Here's how the part is built. I have some questions about the finished solid (model axes, mm). Round coordinates to 2 decimals unless told otherwise and drop trailing zeros. Order: outer loops, then holes, each group sorted by start corner. A loop starts at its lowest first (then second) coordinate and runs counter-clockwise, first axis right, second up. Notation, with made-up numbers: M -20.5,11.5 L 30.5,11.5 A26 ccw 30.5,31.5 Z; hole C -1,-22.5 d10. An arc over 180 degrees is marked long. Write item = value, one per line. Start each with the question number.
Item 1: Please list where these lines run through material, in increasing order: L1, parallel to X at y = 6.5, z = 11.5; L2, parallel to Z at x = 99.5, y = 1; L3, parallel to Y at x = 84.5, z = 0.
Item 2: We'd pull the mould along Y, two halves only. Please class faces 1 (the face through (137.69, -9.76, 2.17)), 2 (the face through (10, -10, -3)): pulls with the +Y half, pulls with the -Y half, needs draft (parallel to the pull), parting line crosses it, or undercut.
Item 3: I want a section at A-A, the plane y = 0. List the corners of the cut face in (x, z) for me.
Item 4: I want a section at B-B, the plane x = 226. List the corners of the cut face in (y, z) for me.
Item 5: I'm going to push flat-ended pins straight in: P1, Ø2, axis at x = 0.5, y = -0.5, coming from the -Z side; P2, Ø8, axis at x = 167, y = -4, coming from the -Z side; P3, Ø5, axis at x = 228.5, z = 4.5, coming from the -Y side. Where does each tip first touch, or does it pass through?
```python
from build123d import *

# Parameters (mm, degrees)
SKETCH1_R           = 15
SKETCH1_R_2         = 10
BOSS_EXTRUDE1_DEPTH = 10
SKETCH1_2_R         = 10
BOSS_EXTRUDE2_DEPTH = 270
CHAMFER1_SIZE       = 1
FILLET1_R           = 1.5
SKETCH2_W           = 3
SKETCH2_H           = 32.549334764
CUT_EXTRUDE1_DEPTH  = 2


with BuildPart() as part:
    # Sketch1 → Boss-Extrude1 (new body)
    with BuildSketch(Plane(origin=(0, 0, 0), x_dir=(0, 0, -1), z_dir=(1, 0, 0))):
        Circle(SKETCH1_R)
        Circle(SKETCH1_R_2, mode=Mode.SUBTRACT)
    extrude(amount=BOSS_EXTRUDE1_DEPTH)

    # Sketch1<2> → Boss-Extrude2 (add)
    with BuildSketch(Plane(origin=(0, 0, 0), x_dir=(0, 0, -1), z_dir=(1, 0, 0))):
        Circle(SKETCH1_2_R)
    extrude(amount=BOSS_EXTRUDE2_DEPTH)

    # Chamfer1
    chamfer1_edges = [part.edges().sort_by_distance(p)[0] for p in [
        (270, 0, 10),
    ]]
    chamfer(chamfer1_edges, length=CHAMFER1_SIZE)

    # Fillet1
    fillet1_edges = [part.edges().sort_by_distance(p)[0] for p in [
        (0, 0, 15),
    ]]
    fillet(fillet1_edges, radius=FILLET1_R)

    # Sketch2 → Cut-Extrude1 (cut)
    with BuildSketch(Plane.ZY):
        Rectangle(SKETCH2_W, SKETCH2_H)
    extrude(amount=-CUT_EXTRUDE1_DEPTH, mode=Mode.SUBTRACT)


solid = part.part
```
Filled in:
q1.L1 = 0 to 10
q1.L2 = -9.95 to 9.95
q1.L3 = -10 to 10
q2.face_1 = parting line crosses it
q2.face_2 = needs draft
q3.outline = M 0,-13.5 A1.5 ccw 1.5,-15 L 10,-15 L 10,-10 L 269,-10 L 270,-9 L 270,9 L 269,10 L 10,10 L 10,15 L 1.5,15 A1.5 ccw 0,13.5 L 0,1.5 L 2,1.5 L 2,-1.5 L 0,-1.5 Z
q4.outline = C 0,0 d20
q5.P1 = -15
q5.P2 = -10
q5.P3 = -9.8
